Work out the finished part from the listing and answer in its coordinate system (mm). A direction names the side the tool comes from. Coordinates: 2 decimals unless noted, no trailing zeros. Write each loop counter-clockwise with the first axis right and the second up, starting at its lowest first coordinate (ties: lowest second). Pieces come first, ordered by that corner, then holes. Notation, with made-up numbers: (52, 70) -> (77, 70) arc R14 ccw to (77, 97) -> close; hole circle Ø7 at (-2.75, -5). An arc over 180 degrees is marked (long way). Write each question's results on one line, items separated by ' | '. Start each with the question number.
from build123d import *

# Parameters (mm, degrees)
M3_CLEARANCE_HOLE1_D = 3.4
SKETCH9_OUTSIDE_W    = 41.38
SKETCH9_OUTSIDE_H    = 41.38
SKETCH9_OUTSIDE_W_2  = 30
SKETCH9_OUTSIDE_H_2  = 10
CUT_EXTRUDE1_DEPTH   = 26.416530054


with BuildPart() as part:
    # Sketch2 → Revolve1 (revolve)
    with BuildSketch(Plane.XY):
        Polygon((0, 0), (-5, 0), (-5, 10), (-15, 10), (-15, 14), (-5, 14), (-5, 20), (0, 20), align=None)
    revolve(axis=Axis((0, 20, 0), (0, -1, 0)))

    # M3 Clearance Hole1 (through all)
    with Locations(Plane(origin=(0, 14, 0), x_dir=(-1, 0, 0), z_dir=(0, 1, 0))):
        with Locations((10, 0), (-10, 0)):
            Hole(M3_CLEARANCE_HOLE1_D / 2)

    # Sketch8 → M6 Tapped Hole1 (revolve, cut)
    with BuildSketch(Plane(origin=(0, 20, 0), x_dir=(0, 0, 1), z_dir=(1, 0, 0))):
        Polygon((0, 0), (0, 20), (3.025, 20), (2.5, 19.475), (2.5, 0.525), (3.025, 0), align=None)
    revolve(axis=Axis((0, 26.35, 0), (0, -1, 0)), mode=Mode.SUBTRACT)

    # Sketch9 outside → Cut-Extrude1 (cut, through all)
    with BuildSketch(Plane(origin=(0, 14, 0), x_dir=(1, 0, 0), z_dir=(0, 1, 0))):
        Rectangle(SKETCH9_OUTSIDE_W, SKETCH9_OUTSIDE_H)
        Rectangle(SKETCH9_OUTSIDE_W_2, SKETCH9_OUTSIDE_H_2, mode=Mode.SUBTRACT)
    extrude(amount=-CUT_EXTRUDE1_DEPTH, mode=Mode.SUBTRACT)


solid = part.part
1. For faces 4 (the face through (1.08, 5.07, 4.88)), 5 (the face through (1.08, 17.04, 4.88)), 6 (the face through (0, 12, -5)), determine the directions among +Z, -Z, +X, -X, +Y, -Y from which every point of the face is accessible in a straight line to the end or side of a thin tool.
2. Determine the mould class of faces 1 (the face through (-3.3, 20, -0.1)), 2 (the face through (-15, 12, 0)), 3 (the face through (-8.43, 11.97, -0.65)) for opening direction X: pulls with the +X half, pulls with the -X half, needs draft (parallel to the pull), parting line crosses it, or undercut.
3. Find the intervals of material crossed by L1, parallel to Z at x = -10, y = 10.9; L2, parallel to Z at x = 0, y = 6.5, in increasing order.
4. Find section A-A on z = 0. Give the vertices of the cut face in (x, y) (3 decimals), and give its area (3 significant figures).
5. Find section B-B on y = 12.5. Give the vertices of the cut face in (x, z), and give its area (3 significant figures).
6. Given pin 1 Ø5 at (x, z) = (-4, 2) entering from -Y; pin 2 Ø1.5 at (x, y) = (-2, 7.5) entering from +Z; pin 3 Ø1.5 at (y, z) = (7.5, 0) entering from +X; pin 4 Ø6 at (x, z) = (-10.5, 3) entering from +Y, each flat-ended and moving along its own axis, determine where each tip first touches the part or whether it passes through.
7. Find section D-D on x = 4. Give the vertices of the cut face in (y, z), and give its area (3 significant figures).
8. Find section C-C on x = 11. Give the vertices of the cut face in (y, z), and give its area (3 significant figures).
Ans:
1) face 4: -Y | face 5: +Y | face 6: -Z, +X, -X, +Y, -Y
2) face 1: needs draft | face 2: pulls with the -X half | face 3: undercut
3) L1: z = -5 to -1.7, 1.7 to 5 | L2: z = -5 to -2.5, 2.5 to 5
4) outline: (-15, 10) -> (-11.7, 10) -> (-11.7, 14) -> (-15, 14) -> close; (-8.3, 10) -> (-5, 10) -> (-5, 0) -> (-3.025, 0) -> (-2.5, 0.525) -> (-2.5, 19.475) -> (-3.025, 20) -> (-5, 20) -> (-5, 14) -> (-8.3, 14) -> close; (2.5, 0.525) -> (3.025, 0) -> (5, 0) -> (5, 10) -> (8.3, 10) -> (8.3, 14) -> (5, 14) -> (5, 20) -> (3.025, 20) -> (2.5, 19.475) -> close; (11.7, 10) -> (15, 10) -> (15, 14) -> (11.7, 14) -> close | area: 152 mm²
5) outline: (-14.14, -5) -> (14.14, -5) arc R15 ccw to (14.14, 5) -> (-14.14, 5) arc R15 ccw to start; hole circle Ø3.4 at (-10, 0); hole circle Ø5 at (0, 0); hole circle Ø3.4 at (10, 0) | area: 257 mm²
6) pin 1: stops at y = 0 | pin 2: stops at z = 4.84 | pin 3: stops at x = 5 | pin 4: stops at y = 14
7) outline: (0, -3) -> (10, -3) -> (10, -5) -> (14, -5) -> (14, -3) -> (20, -3) -> (20, 3) -> (14, 3) -> (14, 5) -> (10, 5) -> (10, 3) -> (0, 3) -> close | area: 136 mm²
8) outline: (10, -5) -> (14, -5) -> (14, -1.37) -> (10, -1.37) -> close; (10, 1.37) -> (14, 1.37) -> (14, 5) -> (10, 5) -> close | area: 29.0 mm²
